Study the drawing (mm; zero at the part's minimum x, y, z) and answer. A direction names the side the tool comes from. Round coordinates to 2 decimals unless told otherwise and drop trailing zeros. Loops run counter-clockwise (first coordinate to the right, second up) from the corner with the lowest first, then second, coordinate; pieces in that order, holes last. Notation, with made-up numbers: M -20.5,-14.75 L 27.5,-14.75 A21 cw 27.5,2.25 Z; hole C 79,52.5 d9. An arc over 180 degrees is marked long. Put each result on its own line as item: value. Start each with the question number.
(1) Straight lines are drawn through the part: line 1 (Z direction, x = 6, y = 14.5); line 2 (X direction, y = 20, z = 4); line 3 (Y direction, x = 56.5, z = 7.5). For each, find the intervals that lie inside material, in ascending order.
(2) Section A-A, the plane x = 66 is taken. Determine the outline of the cut face in (y, z), then the cut area to 3 significant figures.
(3) Section D-D, the plane y = 7 is taken. Determine the outline of the cut face in (x, z), then the cut area to 3 significant figures.
(4) Section C-C, the plane z = 5.75 is taken. Determine the outline of the cut face in (x, y), then the cut area to 3 significant figures.
(5) Flat-ended cylindrical pins translate along their axes: P1, Ø1.8, axis at x = 6, z = 5, coming from the -Y side; P2, Ø3, axis at x = 63, z = 4.5, coming from the +Y side; P3, Ø3, axis at x = 4.5, z = 7, coming from the -Y side; P4, Ø8, axis at x = 60.5, y = 5, coming from the -Z side. Find the tip coordinate at first contact, or state that the pin passes through.
(6) Which of the six approach directions +Z, -Z, +X, -X, +Y, -Y give full straight-line access (tool end or side, diameter ignored) to the marked faces 1, 2 and 3?
(7) Section B-B, the plane y = 21.5 is taken. Count the separate pieces of the cut face and the enclosed holes in it, then the cut area to 3 significant figures.
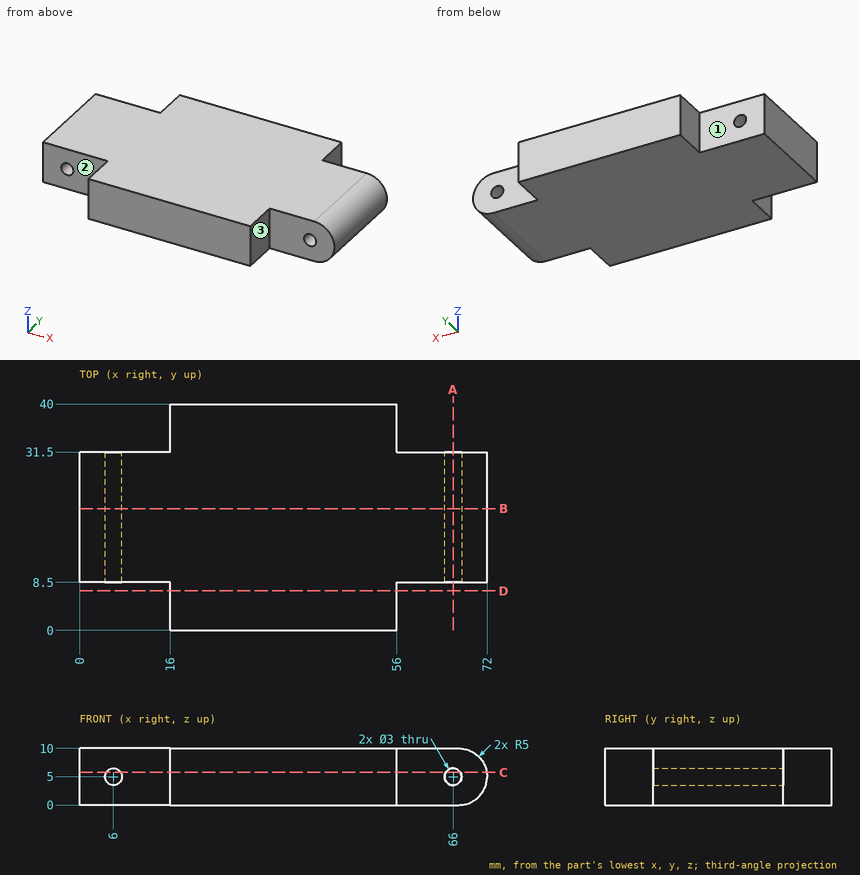
Recorded:
1. line 1: z = 0 to 3.5, 6.5 to 10
1. line 2: x = 0 to 4.88, 7.12 to 64.88, 67.12 to 71.9
1. line 3: y = 8.5 to 31.5
2. outline: M 8.5,0 L 31.5,0 L 31.5,3.5 L 8.5,3.5 Z; M 8.5,6.5 L 31.5,6.5 L 31.5,10 L 8.5,10 Z
2. area: 161 mm²
3. outline: M 16,0 L 56,0 L 56,10 L 16,10 Z
3. area: 400 mm²
4. outline: M 0,8.5 L 4.7,8.5 L 4.7,31.5 L 0,31.5 Z; M 7.3,8.5 L 16,8.5 L 16,0 L 56,0 L 56,8.5 L 64.7,8.5 L 64.7,31.5 L 56,31.5 L 56,40 L 16,40 L 16,31.5 L 7.3,31.5 Z; M 67.3,8.5 L 71.94,8.5 L 71.94,31.5 L 67.3,31.5 Z
4. area: 2,220 mm²
5. P1: passes through
5. P2: stops at y = 31.5
5. P3: stops at y = 8.5
5. P4: stops at z = 0
6. face 1: +Z, -Z, -X, +Y
6. face 2: +Z, -Z, -X, -Y
6. face 3: +Z, -Z, +X, -Y
7. separate pieces: 1
7. enclosed holes: 2
7. area: 695 mm²
